Check sheet for the modelled part. Datum: model origin and axes. Units: mm. Face numbers are marked on the shaded views. A direction names the side the tool comes from. Round coordinates to 2 decimals unless told otherwise and drop trailing zeros. Write each loop counter-clockwise with the first axis right and the second up, starting at its lowest first coordinate (ties: lowest second). Pieces come first, ordered by that corner, then holes.
Item 1: Release check for a two-part mould opening along X. For the marked faces 4, 5, 6 and 7 record: pulls with the +X half, pulls with the -X half, needs draft (parallel to the pull), parting line crosses it, or undercut.
Item 2: Section check A-A, the plane y = -9. Record the cut outline in (x, z).
Item 3: Material ranges on line 1 along X through (y, z) = (-13, 2); line 2 along X through (y, z) = (-22, 1.5); line 3 along Y through (x, z) = (7.5, 2.25), recorded low to high.
Item 4: Section check D-D, the plane y = 24. Record the cut outline in (x, z), plus the area to 3 significant figures.
Item 5: Depth check by flat-ended pin: pin 1 (1.5 mm diameter, centred on x = -24.5, z = 1.5, fed in from +Y); pin 2 (2 mm diameter, centred on y = 29, z = 2, fed in from +X); pin 3 (3.5 mm diameter, centred on y = 20.5, z = 5, fed in from -X); pin 4 (1 mm diameter, centred on x = 9, y = -19, fed in from -Z). Enter the tip coordinate at first touch or a pass-through.
Item 6: Section check B-B, the plane x = 26. Record the cut outline in (y, z), plus the area to 3 significant figures.
Item 7: Set-up check for the marked faces 1, 2 and 3: record each of +Z, -Z, +X, -X, +Y, -Y from which the full face is reachable in a straight line by a thin tool's end or side.
Item 8: Section check C-C, the plane z = 4. State how many separate pieces and enclosed holes the cut face has, plus the area to 3 significant figures.
from build123d import *

# Parameters (mm, degrees)
F0_R     = 11.1
F1_DEPTH = 7
F2_R     = 15.23999
F3_R     = 12.7


# Not quite as in the source:
# - a fillet or chamfer is up to 0.001 mm smaller than in the source, because OpenCascade refuses the exact size


with BuildPart() as f1:
    # F0 (on Top) → F1 (new body)
    with BuildSketch(Plane.XY):
        Polygon((15.24, 40.64), (0, 40.64), (-15.24, 40.64), (-15.24, 8.7988181024), (-42.8152724098, -7.1217728463), (-27.5752724098, -33.5182271537), (0, -17.5976362049), (27.5752724098, -33.5182271537), (42.8152724098, -7.1217728463), (15.24, 8.7988181024), align=None)
        with Locations((-22.4040771959, -12.935)):
            Circle(F0_R, mode=Mode.SUBTRACT)
        with BuildLine():
            ThreePointArc((0, 11.1), (7.8488852712, 7.8488852712), (11.1, 0))
            ThreePointArc((11.1, 0), (-7.8488852712, -7.8488852712), (0, 11.1))
        make_face(mode=Mode.SUBTRACT)
        with Locations((22.4040771959, -12.935)):
            Circle(F0_R, mode=Mode.SUBTRACT)
        with BuildLine():
            ThreePointArc((11.1, 25.87), (7.8488852712, 18.0211147288), (0, 14.77))
            ThreePointArc((0, 14.77), (-11.1, 25.87), (0, 36.97))
            ThreePointArc((0, 36.97), (7.8488852712, 33.7188852712), (11.1, 25.87))
        make_face(mode=Mode.SUBTRACT)
    extrude(amount=F1_DEPTH)

    # F2 (radius 15.24 in the source; OpenCascade refuses exactly that, so slightly less here)
    f2_edges = [f1.edges().sort_by_distance(p)[0] for p in [
        (15.24, 40.64, 3.5),
        (-15.24, 40.64, 3.5),
        (-42.815272, -7.121773, 3.5),
        (-27.575272, -33.518227, 3.5),
        (42.815272, -7.121773, 3.5),
        (27.575272, -33.518227, 3.5),
    ]]
    fillet(f2_edges, radius=F2_R)

    # F3
    f3_edges = [f1.edges().sort_by_distance(p)[0] for p in [
        (15.24, 8.798818, 3.5),
        (0, -17.597636, 3.5),
        (-15.24, 8.798818, 3.5),
    ]]
    fillet(f3_edges, radius=F3_R)


solid = f1.part
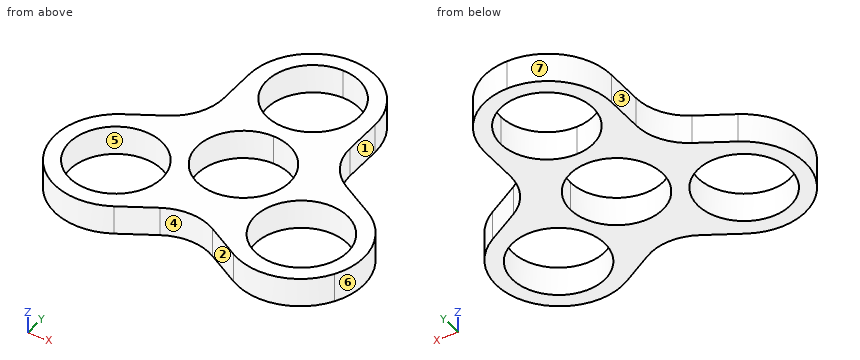
Values found:
1. face 4: undercut
1. face 5: undercut
1. face 6: pulls with the +X half
1. face 7: pulls with the -X half
2. outline: (-36.78, 0) - (-32.78, 0) - (-32.78, 7) - (-36.78, 7) - close; (-12.02, 0) - (-6.5, 0) - (-6.5, 7) - (-12.02, 7) - close; (6.5, 0) - (12.02, 0) - (12.02, 7) - (6.5, 7) - close; (32.78, 0) - (36.78, 0) - (36.78, 7) - (32.78, 7) - close
3. line 1: x = -37.23 to -33.5, -11.3 to 11.3, 33.5 to 37.23
3. line 2: x = -34.07 to -28.81, -16 to -7.63, 7.63 to 16, 28.81 to 34.07
3. line 3: y = -21.93 to -8.18, 8.18 to 17.69, 34.05 to 38.67
4. outline: (-15.24, 0) - (-10.94, 0) - (-10.94, 7) - (-15.24, 7) - close; (10.94, 0) - (15.24, 0) - (15.24, 7) - (10.94, 7) - close
4. area: 60.2 mm2
5. pin 1: stops at y = 3.89
5. pin 2: stops at x = 15.02
5. pin 3: stops at x = -15.24
5. pin 4: stops at z = 0
6. outline: (-27.4, 0) - (-23.44, 0) - (-23.44, 7) - (-27.4, 7) - close; (-2.43, 0) - (2.59, 0) - (2.59, 7) - (-2.43, 7) - close
6. area: 62.9 mm2
7. face 1: +Z, -Z, +X, +Y
7. face 2: +Z, -Z, -Y
7. face 3: +Z, -Z, -X, +Y
8. separate pieces: 1
8. enclosed holes: 4
8. area: 1,490 mm2
